from build123d import *

# Parameters (mm, degrees)
SKETCH_1_W               = 205
SKETCH_1_H               = 118
SKETCH_1_R               = 8.5
SKETCH_1_R_2             = 7.5
SKETCH_1_R_3             = 2.5
EXTRUDE_1_DEPTH          = 5
SKETCH_2_W               = 5
SKETCH_2_H               = 20
EXTRUDE_2_DEPTH          = 5
PATTERN_LINEAR_2_COUNT   = 3
PATTERN_LINEAR_2_PITCH   = 40
MIRROR_2_COPY_1_SKETCH_W = 5
MIRROR_2_COPY_1_SKETCH_H = 20
MIRROR_2_COPY_1_DEPTH    = 5
MIRROR_2_COPY_2_SKETCH_W = 5
MIRROR_2_COPY_2_SKETCH_H = 20
MIRROR_2_COPY_2_DEPTH    = 5
SKETCH_3_W               = 20
SKETCH_3_H               = 5
EXTRUDE_3_DEPTH          = 5
PATTERN_LINEAR_3_COUNT   = 3
PATTERN_LINEAR_3_PITCH   = 40
PATTERN_LINEAR_4_COUNT   = 3
PATTERN_LINEAR_4_PITCH   = 40
SKETCH_5_W               = 5
SKETCH_5_H               = 20
CUT_EXTRUDE_1_DEPTH      = 5
PATTERN_LINEAR_5_COUNT   = 2
PATTERN_LINEAR_5_PITCH   = 40
SKETCH_5_3_W             = 20
SKETCH_5_3_H             = 5
CUT_EXTRUDE_2_DEPTH      = 5
PATTERN_LINEAR_6_COUNT   = 2
PATTERN_LINEAR_6_PITCH   = 40
SKETCH_6_W               = 5
SKETCH_6_H               = 5
CUT_EXTRUDE_3_DEPTH      = 5


with BuildPart() as part:
    # 스케치1 → 보스-돌출1 (new body)
    with BuildSketch(Plane.XY):
        Rectangle(SKETCH_1_W, SKETCH_1_H)
        with Locations((20.971625496, 2)):
            Circle(SKETCH_1_R, mode=Mode.SUBTRACT)
        with Locations((-49.5, 4)):
            Circle(SKETCH_1_R_2, mode=Mode.SUBTRACT)
        with Locations((-5.028374504, 2)):
            Circle(SKETCH_1_R_3, mode=Mode.SUBTRACT)
        with Locations((46.971625496, 2)):
            Circle(SKETCH_1_R_3, mode=Mode.SUBTRACT)
        with Locations((20.971625496, -34)):
            Circle(SKETCH_1_R_2, mode=Mode.SUBTRACT)
    extrude(amount=EXTRUDE_1_DEPTH)

    # 스케치2 → 보스-돌출2 (add)
    with BuildSketch(Plane.XY.offset(5)):
        with Locations((105, -49)):
            Rectangle(SKETCH_2_W, SKETCH_2_H)
    extrude_2 = extrude(amount=-EXTRUDE_2_DEPTH)

    # 선형 패턴2: 보스-돌출2 ×3
    with Locations(*[(0, i * PATTERN_LINEAR_2_PITCH, 0) for i in range(1, PATTERN_LINEAR_2_COUNT)]):
        add(extrude_2)

    # 대칭 복사2: 보스-돌출2 across plane
    add(extrude_2.mirror(Plane(origin=(0, 0, 0), x_dir=(0, 0, 1), z_dir=(1, 0, 0))))

    # 대칭 복사2 copy 1 sketch → 대칭 복사2 copy 1 (add)
    with BuildSketch(Plane(origin=(0, 40, 5), x_dir=(-1, 0, 0), z_dir=(0, 0, 1))):
        with Locations((105, 49)):
            Rectangle(MIRROR_2_COPY_1_SKETCH_W, MIRROR_2_COPY_1_SKETCH_H)
    extrude(amount=-MIRROR_2_COPY_1_DEPTH)

    # 대칭 복사2 copy 2 sketch → 대칭 복사2 copy 2 (add)
    with BuildSketch(Plane(origin=(0, 80, 5), x_dir=(-1, 0, 0), z_dir=(0, 0, 1))):
        with Locations((105, 49)):
            Rectangle(MIRROR_2_COPY_2_SKETCH_W, MIRROR_2_COPY_2_SKETCH_H)
    extrude(amount=-MIRROR_2_COPY_2_DEPTH)

    # 스케치3 → 보스-돌출3 (add)
    with BuildSketch(Plane.XY.offset(5)):
        with Locations((0, 61.5)):
            Rectangle(SKETCH_3_W, SKETCH_3_H)
    extrude_3 = extrude(amount=-EXTRUDE_3_DEPTH)

    # 선형 패턴3: 보스-돌출3 ×3
    with Locations(*[(i * PATTERN_LINEAR_3_PITCH, 0, 0) for i in range(1, PATTERN_LINEAR_3_COUNT)]):
        add(extrude_3)

    # 선형 패턴4: 보스-돌출3 ×3
    with Locations(*[(-i * PATTERN_LINEAR_4_PITCH, 0, 0) for i in range(1, PATTERN_LINEAR_4_COUNT)]):
        add(extrude_3)

    # 스케치5 → 컷-돌출1 (cut)
    with BuildSketch(Plane.XY.offset(5)):
        with Locations((73.471625496, -29)):
            Rectangle(SKETCH_5_W, SKETCH_5_H)
        with Locations((-31.528374504, -29)):
            Rectangle(SKETCH_5_W, SKETCH_5_H)
    cut_extrude_1 = extrude(amount=-CUT_EXTRUDE_1_DEPTH, mode=Mode.SUBTRACT)

    # 선형 패턴5: 컷-돌출1 ×2
    with Locations(*[(0, i * PATTERN_LINEAR_5_PITCH, 0) for i in range(1, PATTERN_LINEAR_5_COUNT)]):
        add(cut_extrude_1, mode=Mode.SUBTRACT)

    # 스케치5<3> → 컷-돌출2 (cut)
    with BuildSketch(Plane.XY.offset(5)):
        with Locations((40.971625496, 28.5)):
            Rectangle(SKETCH_5_3_W, SKETCH_5_3_H)
    cut_extrude_2 = extrude(amount=-CUT_EXTRUDE_2_DEPTH, mode=Mode.SUBTRACT)

    # 선형 패턴6: 컷-돌출2 ×2
    with Locations(*[(-i * PATTERN_LINEAR_6_PITCH, 0, 0) for i in range(1, PATTERN_LINEAR_6_COUNT)]):
        add(cut_extrude_2, mode=Mode.SUBTRACT)

    # 스케치6 → 컷-돌출3 (cut)
    with BuildSketch(Plane.XY.offset(5)):
        with Locations((73.471625496, 28.5)):
            Rectangle(SKETCH_6_W, SKETCH_6_H)
        with Locations((-31.528374504, 28.5)):
            Rectangle(SKETCH_6_W, SKETCH_6_H)
    extrude(amount=-CUT_EXTRUDE_3_DEPTH, mode=Mode.SUBTRACT)


solid = part.part
Could you check a few things on this model? Use its own coordinates, in mm. A direction names the side the tool comes from. Coordinates: 2 decimals unless noted, no trailing zeros. Write each loop counter-clockwise with the first axis right and the second up, starting at its lowest first coordinate (ties: lowest second). Pieces come first, ordered by that corner, then holes. Notation, with made-up numbers: (-1.75, -4.5) - (13.25, -4.5) arc R27 cw to (13.25, 11.5) - close; hole circle Ø2 at (17.25, -5.75). An arc over 180 degrees is marked (long way). Put each result on its own line as item: value. Start each with the question number.
Q1. I'm going to push flat-ended pins straight in: P1, Ø1.5, axis at x = -104.5, z = 1.5, coming from the +Y side; P2, Ø2.5, axis at y = 62.5, z = 1.5, coming from the -X side; P3, Ø10, axis at x = 21, y = 22.5, coming from the -Z side; P4, Ø2.5, axis at x = -93.5, z = 2, coming from the +Y side. Where does each tip first touch, or does it pass through?
Q2. I want a section at A-A on y = -34. Write out the boundary of the cut face in (x, z), plus the area to 3 significant figures.
Q3. Which directions (+Z, -Z, +X, -X, +Y, -Y) give clear straight access to the entire face, cutting with the end or side of a thin tool? Please do faces 1 (the flat face through (105, 41, 3)), 2 (the flat face through (102.5, -29, 2)), 3 (the flat face through (30, 61, 3)), 4 (the flat face through (41, 26, 3)).
Q4. Please list where these lines run through material, in increasing order: L1, parallel to X at y = 14, z = 4.2; L2, parallel to Y at x = -1, z = 3.3; L3, parallel to X at y = -2, z = 1.25.
Q5. I want a section at C-C on x = 60. Write out the boundary of the cut face in (y, z).
Q6. I want a section at B-B on z = 2.95. Count the separate pieces of the cut face and the enclosed holes in it, plus the area to 3 significant figures.
Q7. Thinking about a two-plate mould opening in X: for faces 5 (the flat face through (-9.028, 28, 3)), 6 (the cylindrical face through (-2.72, 1.04, 2.46)), 7 (the flat face through (107.5, -9, 3)), 8 (the flat face through (-105, 21, 3)), which applies, pulls with the +X half, pulls with the -X half, needs draft (parallel to the pull), parting line crosses it, or undercut?
Checks:
1. P1: y = 41
1. P2: x = -90
1. P3: z = 0
1. P4: y = 59
2. outline: (-102.5, 0) - (-34.03, 0) - (-34.03, 5) - (-102.5, 5) - close; (-29.03, 0) - (13.47, 0) - (13.47, 5) - (-29.03, 5) - close; (28.47, 0) - (70.97, 0) - (70.97, 5) - (28.47, 5) - close; (75.97, 0) - (102.5, 0) - (102.5, 5) - (75.97, 5) - close
2. area: 900 mm²
3. face 1: +Z, -Z, +X, +Y
3. face 2: +Z, -Z, +X
3. face 3: +Z, -Z, +Y
3. face 4: +Z, -Z
4. L1: -102.5 to -34.03, -29.03 to 70.97, 75.97 to 102.5
4. L2: -59 to 26, 31 to 64
4. L3: -107.5 to -54, -45 to 13.47, 28.47 to 107.5
5. outline: (-59, 0) - (59, 0) - (59, 5) - (-59, 5) - close
6. separate pieces: 1
6. enclosed holes: 13
6. area: 24,000 mm²
7. face 5: undercut
7. face 6: undercut
7. face 7: pulls with the +X half
7. face 8: needs draft
